```python
from build123d import *

# Parameters (mm, degrees)
SKETCH1_W           = 41.507340187
SKETCH1_H           = 36.387640449
BOSS_EXTRUDE1_DEPTH = 12.7
SKETCH2_R           = 2.899735459
CUT_EXTRUDE1_DEPTH  = 99.974975464


with BuildPart() as part:
    # Sketch1 → Boss-Extrude1 (new body)
    with BuildSketch(Plane(origin=(0, 0, 0), x_dir=(0, 0, -1), z_dir=(1, 0, 0))):
        with Locations((20.753670094, 18.193820225)):
            Rectangle(SKETCH1_W, SKETCH1_H)
        Polygon((41.507340187, 0), (0, 0), (0, -40.754157303), (89.29644131, -40.754157303), (89.29644131, 0), align=None)
    extrude(amount=BOSS_EXTRUDE1_DEPTH)

    # Sketch2 → Cut-Extrude1 (cut, through all)
    with BuildSketch(Plane(origin=(12.7, 0, 0), x_dir=(0, 0, -1), z_dir=(1, 0, 0))):
        with Locations((19.12019242, 24.225046644)):
            Circle(SKETCH2_R)
    cut_extrude1 = extrude(amount=-CUT_EXTRUDE1_DEPTH, mode=Mode.SUBTRACT)

    # Mirror1: Cut-Extrude1 across plane
    add(cut_extrude1.mirror(Plane.ZX), mode=Mode.SUBTRACT)

    # Mirror2: part across plane


with BuildPart() as part_1:
    add(part.part)
    add(part.part.mirror(Plane(origin=(12.7, 0, -89.29644131), x_dir=(1, 0, 0), z_dir=(0, 0, -1))))


solid = part_1.part
```
Geometry check sheet. Reference: the model listing, model coordinates, mm. A direction names the side the tool comes from. Coordinates: 2 decimals unless noted, no trailing zeros. Loops run counter-clockwise (first coordinate to the right, second up) from the corner with the lowest first, then second, coordinate; pieces in that order, holes last. Notation, with made-up numbers: (52, 45) -> (60, 45) arc R18 ccw to (60, 51) -> close; hole circle Ø7 at (45, 71). An arc over 180 degrees is marked (long way). Put each result on its own line as item: value.
1) Gauge pin test, flat ends, axial feed: pin 1 Ø5 at (y, z) = (-24.23, -159.47) entering from +X; pin 2 Ø6 at (x, z) = (8, -110.5) entering from +Y. Record the tip position at first contact, or that the pin passes through.
Result set:
pin 1: passes through
pin 2: stops at y = 0
2) Release check for a two-part mould opening along Y. For faces 3 (the flat face through (6, 0, -89)), 4 (the cylindrical face through (6.44, 24.35, -162.37)), 5 (the flat face through (12.7, -10, -91)) record: released by +Y, released by -Y, zero draft, split by the parting line, or undercut.
Result set:
face 3: released by +Y
face 4: undercut
face 5: zero draft
3) Thickness scan on line 1 (Z direction, x = 4.5, y = 15); line 2 (Y direction, x = 9, z = -78); line 3 (Z direction, x = 4, y = -22). Record the ranges inside material, lowest first.
Result set:
line 1: z = -178.59 to -137.09, -41.51 to 0
line 2: y = -40.75 to 0
line 3: z = -178.59 to -161.33, -157.61 to -20.98, -17.26 to 0
4) Cross-section at C-C on z = -67. Record the boundary of the cut face in (x, y), plus the area to 3 significant figures.
Result set:
outline: (0, -40.75) -> (12.7, -40.75) -> (12.7, 0) -> (0, 0) -> close
area: 518 mm^2
5) Cross-section at B-B on x = 6. Record the boundary of the cut face in (y, z).
Result set:
outline: (-40.75, -178.59) -> (36.39, -178.59) -> (36.39, -137.09) -> (0, -137.09) -> (0, -41.51) -> (36.39, -41.51) -> (36.39, 0) -> (-40.75, 0) -> close; hole circle Ø5.8 at (-24.23, -159.47); hole circle Ø5.8 at (-24.23, -19.12); hole circle Ø5.8 at (24.23, -159.47); hole circle Ø5.8 at (24.23, -19.12)
6) Tool access check on faces 1 (the flat face through (6, 18, -41.507)), 2 (the flat face through (6, 36.388, -20)). Record the directions out of +Z, -Z, +X, -X, +Y, -Y that give a thin tool (end or side, any length) a straight path to the whole face; none if there is none.
Result set:
face 1: +X, -X, +Y
face 2: +Z, -Z, +X, -X, +Y
7) Cross-section at A-A on y = 6. Record the boundary of the cut face in (x, z).
Result set:
outline: (0, -178.59) -> (12.7, -178.59) -> (12.7, -137.09) -> (0, -137.09) -> close; (0, -41.51) -> (12.7, -41.51) -> (12.7, 0) -> (0, 0) -> close
